from build123d import *
from OCP.BRepFilletAPI import BRepFilletAPI_MakeChamfer

# Parameters (mm, degrees)
SKIZZE1_W               = 24.9
SKIZZE1_H               = 24.05
SKIZZE1_R               = 1.1
PCB_DEPTH               = 0.9
BOSS_EXTRUDE1_DEPTH     = 0.05
SKIZZE3_W               = 20.8
SKIZZE3_H               = 5.5
CONNECTOR_CLOSED_DEPTH  = 2.4
ESQUISSE1_W             = 1.22
ESQUISSE1_H             = 0.8
STATUS_LED_DEPTH        = 0.2
ESQUISSE3_W             = 18.8
ESQUISSE3_H             = 1.1
ENL_V_MAT_EXTRU_1_DEPTH = 0.5
FILLET1_R               = 0.5
CHAMFER1_SIZE           = 0.05
CHAMFER1_SIZE_2         = 0.5


with BuildPart() as part:
    # Skizze1 → PCB (new body)
    with BuildSketch(Plane(origin=(0, 0, 0), x_dir=(1, 0, 0), z_dir=(0, 1, 0))):
        with Locations((-0.3, 1.855)):
            Rectangle(SKIZZE1_W, SKIZZE1_H)
        with Locations(Location((-10.65, 11.78, 0), (0, 0, 270))):
            Circle(SKIZZE1_R, mode=Mode.SUBTRACT)
        with Locations(Location((10.35, 11.78, 0), (0, 0, 270))):
            Circle(SKIZZE1_R, mode=Mode.SUBTRACT)
        with Locations(Location((-10.45, -0.72, 0), (0, 0, 270))):
            Circle(SKIZZE1_R, mode=Mode.SUBTRACT)
        with Locations(Location((10.05, -0.72, 0), (0, 0, 270))):
            Circle(SKIZZE1_R, mode=Mode.SUBTRACT)
    extrude(amount=-PCB_DEPTH)

    # Sketch4 → Boss-Extrude1 (add)
    with BuildSketch(Plane(origin=(0, 0, 0), x_dir=(1, 0, 0), z_dir=(0, 1, 0))):
        Polygon((-4.3, 4.3), (-3, 4.3), (-3, 4.8), (-4.8, 4.8), (-4.8, -4.8), (4.8, -4.8), (4.8, 4.8), (3, 4.8), (3, 4.3), (4.3, 4.3), (4.3, -4.3), (-4.3, -4.3), align=None)
    extrude(amount=BOSS_EXTRUDE1_DEPTH)

    # Skizze3 → Connector_closed (add)
    with BuildSketch(Plane.XZ.offset(0.9)):
        with Locations((0, 7.42)):
            Rectangle(SKIZZE3_W, SKIZZE3_H)
    extrude(amount=CONNECTOR_CLOSED_DEPTH)

    # Esquisse1 → Status LED (add)
    with BuildSketch(Plane(origin=(0, 0, 0), x_dir=(1, 0, 0), z_dir=(0, 1, 0))):
        with Locations((7.74, 8.88)):
            Rectangle(ESQUISSE1_W, ESQUISSE1_H)
    extrude(amount=STATUS_LED_DEPTH)

    # Esquisse3 → Enlèv. mat.-Extru.1 (cut)
    with BuildSketch(Plane.XY.offset(10.17)):
        with Locations((0, -1.95)):
            Rectangle(ESQUISSE3_W, ESQUISSE3_H)
    extrude(amount=-ENL_V_MAT_EXTRU_1_DEPTH, mode=Mode.SUBTRACT)

    # Fillet1
    fillet1_edges = [part.edges().sort_by_distance(p)[0] for p in [
        (-4.8, 0.025, -4.8),
        (-4.8, 0.025, 4.8),
        (4.8, 0.025, 4.8),
        (4.8, 0.025, -4.8),
    ]]
    fillet(fillet1_edges, radius=FILLET1_R)

    # Chamfer1
    chamfer1_edges_1 = [part.edges().sort_by_distance(p)[0] for p in [
        (3.65, 0.05, -4.8),
    ]]
    chamfer1_side_1 = [part.faces().sort_by_distance(p)[0] for p in [
        (3.65, 0.049, -4.8),
    ]]
    chamfer1_edges_2 = [part.edges().sort_by_distance(p)[0] for p in [
        (4.8, 0.05, 0),
    ]]
    chamfer1_side_2 = [part.faces().sort_by_distance(p)[0] for p in [
        (4.8, 0.049, 0),
    ]]
    chamfer1_edges_3 = [part.edges().sort_by_distance(p)[0] for p in [
        (0, 0.05, 4.8),
    ]]
    chamfer1_side_3 = [part.faces().sort_by_distance(p)[0] for p in [
        (0, 0.049, 4.8),
    ]]
    chamfer1_edges_4 = [part.edges().sort_by_distance(p)[0] for p in [
        (-4.8, 0.05, 0),
    ]]
    chamfer1_side_4 = [part.faces().sort_by_distance(p)[0] for p in [
        (-4.8, 0.049, 0),
    ]]
    chamfer1_edges_5 = [part.edges().sort_by_distance(p)[0] for p in [
        (-3.65, 0.05, -4.8),
    ]]
    chamfer1_side_5 = [part.faces().sort_by_distance(p)[0] for p in [
        (-3.65, 0.049, -4.8),
    ]]
    chamfer1_edges_6 = [part.edges().sort_by_distance(p)[0] for p in [
        (4.653553391, 0.05, -4.653553391),
    ]]
    chamfer1_side_6 = [part.faces().sort_by_distance(p)[0] for p in [
        (4.653553391, 0.049, -4.653553391),
    ]]
    chamfer1_edges_7 = [part.edges().sort_by_distance(p)[0] for p in [
        (4.653553391, 0.05, 4.653553391),
    ]]
    chamfer1_side_7 = [part.faces().sort_by_distance(p)[0] for p in [
        (4.653553391, 0.049, 4.653553391),
    ]]
    chamfer1_edges_8 = [part.edges().sort_by_distance(p)[0] for p in [
        (-4.653553391, 0.05, 4.653553391),
    ]]
    chamfer1_side_8 = [part.faces().sort_by_distance(p)[0] for p in [
        (-4.653553391, 0.049, 4.653553391),
    ]]
    chamfer1_edges_9 = [part.edges().sort_by_distance(p)[0] for p in [
        (-4.653553391, 0.05, -4.653553391),
    ]]
    chamfer1_side_9 = [part.faces().sort_by_distance(p)[0] for p in [
        (-4.653553391, 0.049, -4.653553391),
    ]]
    chamfer1 = BRepFilletAPI_MakeChamfer(part.part.solid().wrapped)
    for e in chamfer1_edges_1:
        chamfer1.Add(CHAMFER1_SIZE - 0.0001, CHAMFER1_SIZE_2 - 0.0001, e.wrapped, chamfer1_side_1[0].wrapped)
    for e in chamfer1_edges_2:
        chamfer1.Add(CHAMFER1_SIZE - 0.0001, CHAMFER1_SIZE_2 - 0.0001, e.wrapped, chamfer1_side_2[0].wrapped)
    for e in chamfer1_edges_3:
        chamfer1.Add(CHAMFER1_SIZE - 0.0001, CHAMFER1_SIZE_2 - 0.0001, e.wrapped, chamfer1_side_3[0].wrapped)
    for e in chamfer1_edges_4:
        chamfer1.Add(CHAMFER1_SIZE - 0.0001, CHAMFER1_SIZE_2 - 0.0001, e.wrapped, chamfer1_side_4[0].wrapped)
    for e in chamfer1_edges_5:
        chamfer1.Add(CHAMFER1_SIZE - 0.0001, CHAMFER1_SIZE_2 - 0.0001, e.wrapped, chamfer1_side_5[0].wrapped)
    for e in chamfer1_edges_6:
        chamfer1.Add(CHAMFER1_SIZE - 0.0001, CHAMFER1_SIZE_2 - 0.0001, e.wrapped, chamfer1_side_6[0].wrapped)
    for e in chamfer1_edges_7:
        chamfer1.Add(CHAMFER1_SIZE - 0.0001, CHAMFER1_SIZE_2 - 0.0001, e.wrapped, chamfer1_side_7[0].wrapped)
    for e in chamfer1_edges_8:
        chamfer1.Add(CHAMFER1_SIZE - 0.0001, CHAMFER1_SIZE_2 - 0.0001, e.wrapped, chamfer1_side_8[0].wrapped)
    for e in chamfer1_edges_9:
        chamfer1.Add(CHAMFER1_SIZE - 0.0001, CHAMFER1_SIZE_2 - 0.0001, e.wrapped, chamfer1_side_9[0].wrapped)
    add(Compound.cast(chamfer1.Shape()), mode=Mode.REPLACE)  # a hair under: the kernel refuses the full size


solid = part.part
Model file for the job. Use its own axes, mm. A direction names the side the tool comes from. Round coordinates to 2 decimals unless told otherwise and drop trailing zeros. Loops run counter-clockwise (first coordinate to the right, second up) from the corner with the lowest first, then second, coordinate; pieces in that order, holes last.
1. Band-saw the part on B-B, the plane y = -0.3. List the corners of the cut face in (x, z), and give its area (3 significant figures).
Check values:
outline: (-12.75, -13.88) - (12.15, -13.88) - (12.15, 10.17) - (-12.75, 10.17) - close; hole circle Ø2.2 at (-10.65, -11.78); hole circle Ø2.2 at (-10.45, 0.72); hole circle Ø2.2 at (10.05, 0.72); hole circle Ø2.2 at (10.35, -11.78)
area: 584 mm2
2. Band-saw the part on C-C, the plane x = -11. List the corners of the cut face in (y, z), and give its area (3 significant figures).
Check values:
outline: (-0.9, -13.88) - (0, -13.88) - (0, -12.82) - (-0.9, -12.82) - close; (-0.9, -10.74) - (0, -10.74) - (0, -0.23) - (-0.9, -0.23) - close; (-0.9, 1.67) - (0, 1.67) - (0, 10.17) - (-0.9, 10.17) - close
area: 18.1 mm2
3. Tool access for faces 1 (the flat face through (0, -2, 4.67)), 2 (the cylindrical face through (-9.36, -0.44, 0.58)), 3 (the flat face through (10.4, -2, 7)): list every direction of +Z, -Z, +X, -X, +Y, -Y with a clear straight run to the whole face (end or side of a thin tool).
Check values:
face 1: -Z, +X, -X, -Y
face 2: +Y, -Y
face 3: +Z, -Z, +X, -Y
4. Wall check: probe 1 along X at (y, z) = (-0.2, -11.78); probe 2 along X at (y, z) = (-0.6, 0.72); probe 3 along Y at (x, z) = (9.5, -7.5). Give the ranges that are in metal, low to high.
Check values:
probe 1: x = -12.75 to -11.75, -9.55 to 9.25, 11.45 to 12.15
probe 2: x = -12.75 to -11.55, -9.35 to 8.95, 11.15 to 12.15
probe 3: y = -0.9 to 0
5. Mould opens along Y. For faces 4 (the flat face through (-10.4, -2, 7)), 5 (the flat face through (0, -3.3, 7)), 6 (the flat face through (0, -2, 9.67)) say: +Y half, -Y half, draft (parallel to the pull), parting line (faces both ways), or undercut.
Check values:
face 4: draft
face 5: -Y half
face 6: undercut
6. Drop flat-ended pins along their axis: P1, Ø2, axis at x = 3, z = 3.5, coming from the -Y side; P2, Ø0.6, axis at y = -2, z = 10, coming from the +X side; P3, Ø2, axis at x = -8.5, y = -2.5, coming from the -Z side. Give the stop position or say it passes through.
Check values:
P1: stops at y = -0.9
P2: stops at x = 10.4
P3: stops at z = 4.67
7. Band-saw the part on A-A, the plane z = 0.72. Count the separate pieces of the cut face and the enclosed holes in it, and give its area (3 significant figures).
Check values:
separate pieces: 3
enclosed holes: 0
area: 18.5 mm2
